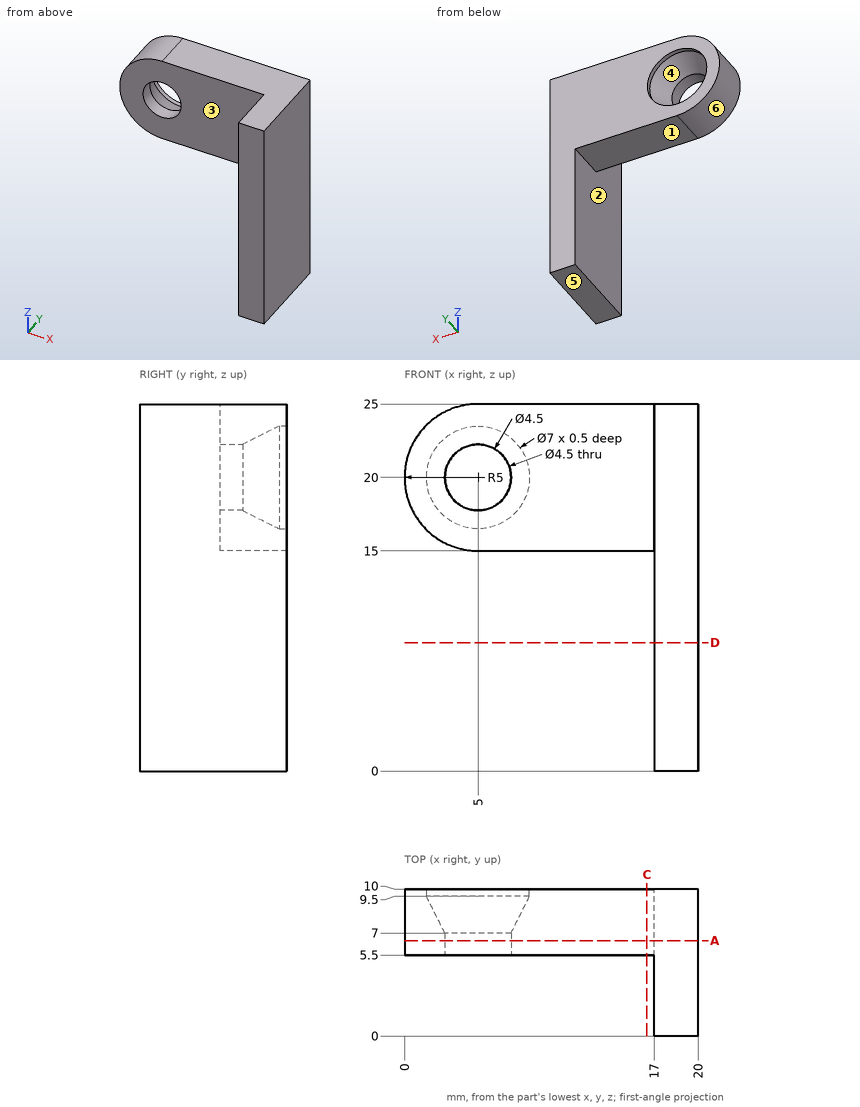
Geometry: see drawing. Coordinates: mm, zero at the bounding-box minimum. A direction names the side the tool comes from. Round coordinates to 2 decimals unless told otherwise and drop trailing zeros. Write each loop counter-clockwise with the first axis right and the second up, starting at its lowest first coordinate (ties: lowest second). Pieces come first, ordered by that corner, then holes. Notation, with made-up numbers: (-36, 80) -> (9, 80) arc R22 ccw to (9, 87) -> close; hole circle Ø3 at (-14.5, 53). An arc over 180 degrees is marked (long way). Answer as CSV lines item,"result".
1. Section A-A (y = 6.5). Return the cut outline in (x, z), plus the area to 3 significant figures.
Geometry says:
outline,"(5, 15) -> (17, 15) -> (17, 0) -> (20, 0) -> (20, 25) -> (5, 25) arc R5 ccw to start; hole circle Ø4.5 at (5, 20)"
area,"218 mm^2"
2. Section D-D (z = 8.75). Return the cut outline in (x, y).
Geometry says:
outline,"(17, 0) -> (20, 0) -> (20, 10) -> (17, 10) -> close"
3. Section C-C (x = 16.5). Return the cut outline in (y, z).
Geometry says:
outline,"(5.5, 15) -> (10, 15) -> (10, 25) -> (5.5, 25) -> close"
4. Contact query for flat-ended pins moving along their axis: P1, Ø5, axis at x = 13, y = 7.5, coming from the -Z side; P2, Ø7, axis at x = 5, z = 20, coming from the -Y side. Output: stop coordinate, or through.
Geometry says:
P1,"stops at z = 15"
P2,"stops at y = 5.5"
5. Reachability of the marked faces 1, 2 and 3 from +Z, -Z, +X, -X, +Y, -Y: full face, straight path, thin tool, end or side. Return the list, or none.
Geometry says:
face 1,"-Z, -X, +Y, -Y"
face 2,"-Z, -X, -Y"
face 3,"+Z, -Z, -X, -Y"
6. Ray query, L1, parallel to Z at x = 5, y = 6.75; L2, parallel to X at y = 6.45, z = 20; L3, parallel to X at y = 1.5, z = 8. Return the intervals inside material, ascending. Write a range as [from, to].
Geometry says:
L1,"z = [15, 17.75], [22.25, 25]"
L2,"x = [0, 2.75], [7.25, 20]"
L3,"x = [17, 20]"
7. Mould query, pull axis X, two halves, no side actions, for the marked faces 4, 5 and 6. Classes: +X half, -X half, draft (parallel to the pull), parting line (faces both ways), or undercut.
Geometry says:
face 4,"undercut"
face 5,"draft"
face 6,"-X half"
